Read the model definition and answer for the solid it produces. Units are mm, in the model's axes. Coordinates: 2 decimals unless noted, no trailing zeros. Loops run counter-clockwise (first coordinate to the right, second up) from the corner with the lowest first, then second, coordinate; pieces in that order, holes last. Notation, with made-up numbers: M 44,21 L 66,21 A20 cw 66,55 Z; hole C -37,50.5 d2. An arc over 180 degrees is marked long. Use one line per item in the form item = value. Start each with the question number.
1. Find the intervals of material crossed by probe 1 along Z at (x, y) = (44.45, -1.5) (1 decimal); probe 2 along X at (y, z) = (-1.7, -63.5) (1 decimal); probe 3 along Z at (x, y) = (2.5, -1.85), in increasing order. Write a range as [from, to].
2. The part is cut by section D-D (x = 19). Give the vertices of the cut face in (y, z).
3. The part is cut by section B-B (x = 12). Give the vertices of the cut face in (y, z).
4. The part is cut by section C-C (z = -42.5). Give the vertices of the cut face in (x, y).
5. The part is cut by section A-A (y = -0.6). Give the number of separate pieces and of enclosed holes in the cut face, plus the area to 3 significant figures.
6. For a pull along Z with two mould halves and no side action, classify faces 1 (the flat face through (3, 0, -5)), 2 (the cylindrical face through (52.386, -1.252, -63.675)), 3 (the cylindrical face through (11.41, -1.25, -53.53)) as released by +Z, released by -Z, zero draft, split by the parting line, or undercut.
from build123d import *

# Parameters (mm, degrees)
F0_R     = 3.175
F1_DEPTH = 2.54
F2_DEPTH = 2.54


with BuildPart() as f1:
    # F0 (on Front) → F1 (new body)
    with BuildSketch(Plane.XZ):
        with BuildLine():
            ThreePointArc((-9.525, 50.8), (-6.7351920908, 44.0648079092), (0, 41.275))
            ThreePointArc((0, 41.275), (6.7351920908, 44.0648079092), (9.525, 50.8))
            ThreePointArc((9.525, 50.8), (0, 60.325), (-9.525, 50.8))
        make_face()
        with BuildLine():
            ThreePointArc((3.175, 50.8), (2.2450640303, 48.5549359697), (0, 47.625))
            ThreePointArc((0, 47.625), (-2.2450640303, 53.0450640303), (3.175, 50.8))
        make_face(mode=Mode.SUBTRACT)
        with BuildLine():
            ThreePointArc((9.525, 50.8), (6.7351920908, 44.0648079092), (0, 41.275))
            Line((0, 41.275), (0, 31.7220508101))
            Line((0, 31.7220508101), (0, 15.875))
            ThreePointArc((0, 15.875), (10.4912828764, 11.9142187578), (15.747456912, 2.0082892734))
            Line((15.747456912, 2.0082892734), (9.525, 50.8))
        make_face()
        with BuildLine():
            Line((0, 31.7220508101), (0, 41.275))
            ThreePointArc((0, 41.275), (-6.7351920908, 44.0648079092), (-9.525, 50.8))
            Line((-9.525, 50.8), (-15.7474568676, 2.0082896216))
            ThreePointArc((-15.7474568676, 2.0082896216), (-10.4912827447, 11.9142188737), (0, 15.875))
            Line((0, 15.875), (0, 31.7220508101))
        make_face()
        with Locations((-3.175, 31.7220508101)):
            Circle(F0_R, mode=Mode.SUBTRACT)
        with BuildLine():
            ThreePointArc((15.747456912, 2.0082892734), (10.4912828764, 11.9142187578), (0, 15.875))
            Line((0, 15.875), (0, 3.175))
            ThreePointArc((0, 3.175), (2.2450640303, 2.2450640303), (3.175, 0))
            ThreePointArc((3.175, 0), (2.2450640303, -2.2450640303), (0, -3.175))
            Line((0, -3.175), (0, -15.875))
            ThreePointArc((0, -15.875), (10.4912827447, -11.9142188737), (15.7474568676, -2.0082896216))
            ThreePointArc((15.7474568676, -2.0082896216), (15.8430821303, -1.006167786), (15.875, 0))
            ThreePointArc((15.875, 0), (15.8430821414, 1.0061676109), (15.747456912, 2.0082892734))
        make_face()
        with BuildLine():
            Line((0, 3.175), (0, 15.875))
            ThreePointArc((0, 15.875), (-10.4912827447, 11.9142188737), (-15.7474568676, 2.0082896216))
            ThreePointArc((-15.7474568676, 2.0082896216), (-15.875, 8.81e-08), (-15.7474568899, -2.0082894468))
            ThreePointArc((-15.7474568899, -2.0082894468), (-10.4912828108, -11.9142188155), (0, -15.875))
            Line((0, -15.875), (0, -3.175))
            ThreePointArc((0, -3.175), (-3.175, 0), (0, 3.175))
        make_face()
        with BuildLine():
            ThreePointArc((-15.7474568899, -2.0082894468), (-15.875, 8.81e-08), (-15.7474568676, 2.0082896216))
            Line((-15.7474568676, 2.0082896216), (-16.0035761028, 0))
            Line((-16.0035761028, 0), (-15.7474568899, -2.0082894468))
        make_face()
        with BuildLine():
            Line((16.0035761028, 0), (15.747456912, 2.0082892734))
            ThreePointArc((15.747456912, 2.0082892734), (15.8430821414, 1.0061676109), (15.875, 0))
            ThreePointArc((15.875, 0), (15.8430821303, -1.006167786), (15.7474568676, -2.0082896216))
            Line((15.7474568676, -2.0082896216), (16.0035761028, 0))
        make_face()
        with BuildLine():
            ThreePointArc((0, -15.875), (-10.4912828108, -11.9142188155), (-15.7474568899, -2.0082894468))
            Line((-15.7474568899, -2.0082894468), (-7.778839662, -64.4920434004))
            ThreePointArc((-7.778839662, -64.4920434004), (-5.8853183801, -58.3175754555), (0, -55.6581573215))
            Line((0, -55.6581573215), (0, -15.875))
        make_face()
        with BuildLine():
            ThreePointArc((15.7474568676, -2.0082896216), (10.4912827447, -11.9142188737), (0, -15.875))
            Line((0, -15.875), (0, -55.6581573215))
            ThreePointArc((0, -55.6581573215), (5.545020135, -57.954979865), (7.8418426785, -63.5))
            Line((7.8418426785, -63.5), (36.5125, -63.5))
            ThreePointArc((36.5125, -63.5), (38.831302744, -57.8933836055), (44.4329150916, -55.5625183871))
            Line((44.4329150916, -55.5625183871), (16.1347817513, -55.6234282624))
            ThreePointArc((16.1347817513, -55.6234282624), (11.3599454256, -53.4750825896), (9.8221310627, -48.4701272399))
            Line((9.8221310627, -48.4701272399), (15.7474568676, -2.0082896216))
        make_face()
        with BuildLine():
            ThreePointArc((0, -55.6581573215), (-5.8853183801, -58.3175754555), (-7.778839662, -64.4920434004))
            ThreePointArc((-7.778839662, -64.4920434004), (-5.0761507437, -69.4772226177), (0.2809454712, -71.3368084216))
            ThreePointArc((0.2809454712, -71.3368084216), (5.6434752937, -68.9447849548), (7.8418426785, -63.5))
            Line((7.8418426785, -63.5), (3.175, -63.5))
            ThreePointArc((3.175, -63.5), (-2.2450640303, -65.7450640303), (0, -60.325))
            Line((0, -60.325), (0, -55.6581573215))
        make_face()
        with BuildLine():
            ThreePointArc((7.8418426785, -63.5), (5.6434752937, -68.9447849548), (0.2809454712, -71.3368084216))
            Line((0.2809454712, -71.3368084216), (44.4319013308, -71.4374793662))
            ThreePointArc((44.4319013308, -71.4374793662), (38.8309447219, -69.1062575781), (36.5125, -63.5))
            Line((36.5125, -63.5), (7.8418426785, -63.5))
        make_face()
        with BuildLine():
            ThreePointArc((36.5125, -63.5), (38.8309447219, -69.1062575781), (44.4319013308, -71.4374793662))
            ThreePointArc((44.4319013308, -71.4374793662), (50.0562575781, -69.1190552781), (52.3875, -63.5))
            ThreePointArc((52.3875, -63.5), (50.0566163945, -57.881302744), (44.4329150916, -55.5625183871))
            ThreePointArc((44.4329150916, -55.5625183871), (38.831302744, -57.8933836055), (36.5125, -63.5))
        make_face()
        with BuildLine():
            ThreePointArc((47.625, -63.5), (44.45, -66.675), (41.275, -63.5))
            ThreePointArc((41.275, -63.5), (44.45, -60.325), (47.625, -63.5))
        make_face(mode=Mode.SUBTRACT)
    extrude(amount=F1_DEPTH)

    # F0 (on Front) → F2 (join)
    with BuildSketch(Plane.XZ):
        with BuildLine():
            ThreePointArc((7.8418426785, -63.5), (5.545020135, -57.954979865), (0, -55.6581573215))
            Line((0, -55.6581573215), (0, -60.325))
            ThreePointArc((0, -60.325), (2.2450640303, -61.2549359697), (3.175, -63.5))
            Line((3.175, -63.5), (7.8418426785, -63.5))
        make_face()
    extrude(amount=F2_DEPTH)


solid = f1.part
Computed values:
q1.probe_1 = [-71.4, -66.7], [-60.3, -55.6]
q1.probe_2 = [-7.9, -3.2], [3.2, 41.3], [47.6, 52.4]
q1.probe_3 = [-71.34, -65.46], [-61.54, -1.96], [1.96, 48.84], [52.76, 59.99]
q2.outline = M -2.54,-71.38 L 0,-71.38 L 0,-55.62 L -2.54,-55.62 Z
q3.outline = M -2.54,-71.36 L 0,-71.36 L 0,-54.1 L -2.54,-54.1 Z; M -2.54,-31.39 L 0,-31.39 L 0,31.39 L -2.54,31.39 Z
q4.outline = M -10.58,-2.54 L 10.58,-2.54 L 10.58,0 L -10.58,0 Z
q5.separate_pieces = 1
q5.enclosed_holes = 5
q5.area = 3,590 mm²
q6.face_1 = zero draft
q6.face_2 = split by the parting line
q6.face_3 = undercut
